Autodesk Inventor part; units mm, degrees
ref_plane "YZ Plane" through (0, 0, 0) normal (1, 0, 0) x (0, 1, 0)
ref_plane "XZ Plane" through (0, 0, 0) normal (0, 1, 0) x (-1, 0, 0)
ref_plane "XY Plane" through (0, 0, 0) normal (0, 0, 1) x (1, 0, 0)
sketch "Sketch1" plane through (0, 0, 0) normal (1, 0, 0) x (0, 1, 0)
  line L0 (0, 0) -> (1, 0)
  line L1 (1, 0) -> (3.2, -0.7529)
  line L2 (3.2, -0.7529) -> (3.2, -1.2529)
  line L3 (3.2, -1.2529) -> (0, -1.2529)
  line L4 (0, -1.2529) -> (0, 0)
  line L5 (0, -2.5059) -> (1, -2.5059)
  line L6 (1, -2.5059) -> (3.2, -1.7529)
  line L7 (3.2, -1.7529) -> (3.2, -1.2529)
  line L8 (0, -1.2529) -> (0, -2.5059)
  line L9 (1, -2.5059) -> (1, -3.0059)
  line L10 (1, -3.0059) -> (0, -3.0059)
  line L11 (0, -3.0059) -> (0, -2.5059)
  line L12 (0, -6.0118) -> (1, -6.0118)
  line L13 (1, -6.0118) -> (3.2, -5.2588)
  line L14 (3.2, -5.2588) -> (3.2, -4.7588)
  line L15 (0, -4.7588) -> (0, -6.0118)
  line L16 (3.2, -4.2588) -> (3.2, -4.7588)
  line L17 (1, -3.5059) -> (3.2, -4.2588)
  line L18 (0, -4.7588) -> (0, -3.5059)
  line L19 (1, -3.5059) -> (1, -3.0059)
  line L20 (0, -3.0059) -> (0, -3.5059)
  line L21 (1, -2.5059) -> (1, 0)
  dimension "d1" = 1
  dimension "d2" = 1
  dimension "d3" = 1
  dimension "d4" = 2.2
  dimension "d10" = 3.5059
extrude "Extrusion2" add sketch "Sketch1" along normal blind 8 contours L0 L21 L3 L4 | L3 L21 L5 L8 | L5 L9 L10 L11 | L10 L19 L17 L16 L14 L13 L12 L15 L18 L20
extrude "Extrusion3" add sketch "Sketch1" along normal up to surface (8 mm away) contours L1 L2 L3 L21 | L3 L7 L6 L21
pattern_linear "Rectangular Pattern1" count 16 spacing 3.5059 along (0, 0, -1) of "Extrusion2"
equation "\"d15\" = d10"
properties part number "bolt-rack"
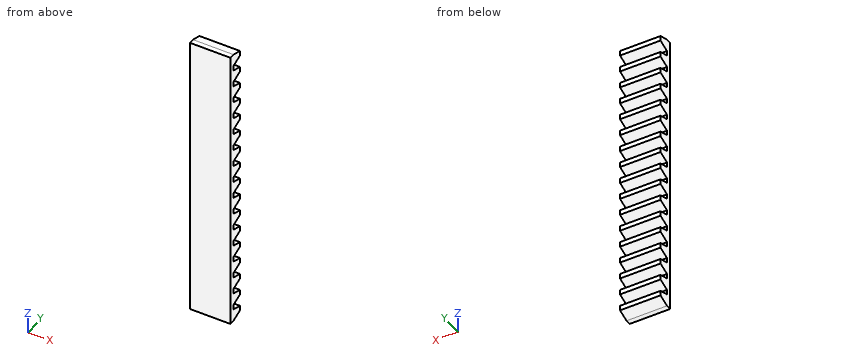
Source: CAD feature listing. Evaluate the final solid. Frame: model axes, mm. Round coordinates to 2 decimals unless told otherwise and drop trailing zeros. Use a Markdown table: item, result. Add a question column.
1. Section query A-A on y = 1.7. Give the number of separate pieces and of enclosed holes in the cut face, then the cut area to 3 significant figures.
2. Contact query for flat-ended pins moving along their axis: P1, Ø0.8, axis at x = 6, z = -17, coming from the +Y side; P2, Ø1, axis at x = 6, y = 2, coming from the +Z side. Output: stop coordinate, or through.
3. Line query: line 1 (Y direction, x = 1, z = -52). Output: solid intervals per line, ascending.
Reported:
| question | item | result |
|---|---|---|
| 1 | separate pieces | 17 |
| 1 | enclosed holes | 0 |
| 1 | area | 276 mm² |
| 2 | P1 | stops at y = 1 |
| 2 | P2 | stops at z = -0.17 |
| 3 | line 1 | y = 0 to 1 |
